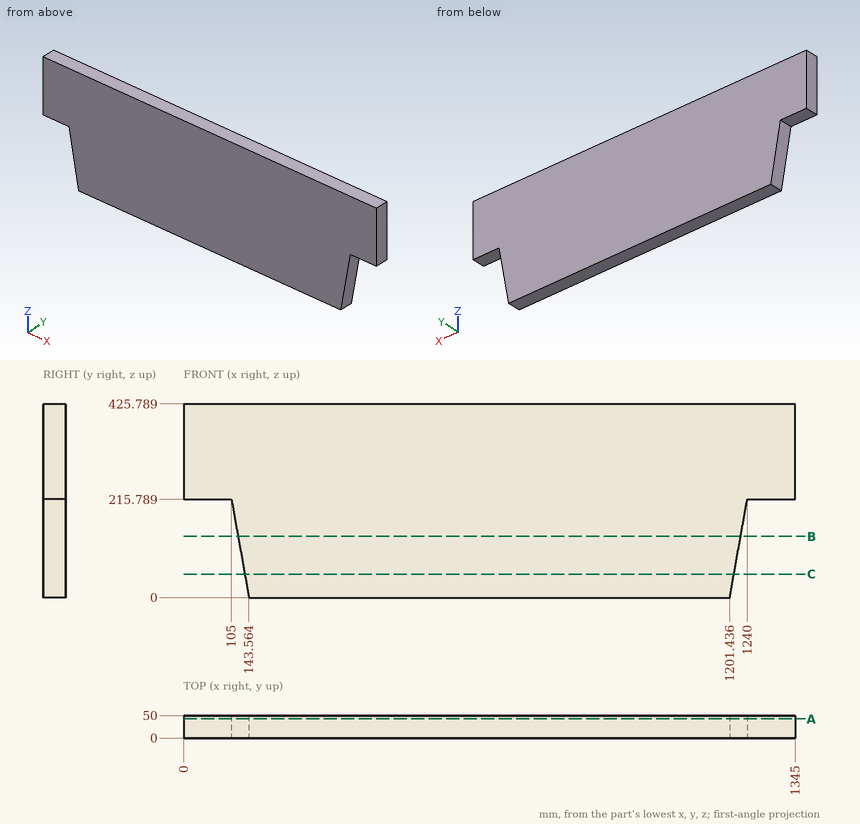
Geometry check sheet. Reference: drawing and pictorial views, mm from the part's lowest x, y, z. Give positions to 0.01 mm unless a question says otherwise; leave off trailing zeros. Loops run counter-clockwise (first coordinate to the right, second up) from the corner with the lowest first, then second, coordinate; pieces in that order, holes last. Notation, with made-up numbers: (-10.5, -19.5) -> (41.5, -19.5) arc R18 ccw to (41.5, -1.5) -> close; hole circle Ø4 at (-4, 49). An arc over 180 degrees is marked (long way). Answer in a Markdown table with one row per item. Add a question column.
1) Cross-section at C-C on z = 51.5. Record the boundary of the cut face in (x, y).
2) Cross-section at A-A on y = 42.5. Record the boundary of the cut face in (x, z) (1 decimal).
3) Cross-section at B-B on z = 134.5. Record the boundary of the cut face in (x, y), and give its area (3 significant figures).
4) Material ranges on probe 1 along Z at (x, y) = (87, 2); probe 2 along X at (y, z) = (34, 24) (1 decimal); probe 3 along X at (y, z) = (18.5, 93), recorded low to high. Write a range as from..to.
5) Gauge pin test, flat ends, axial feed: P1, Ø10, axis at y = 33, z = 86, coming from the +X side; P2, Ø15, axis at x = 1307.5, y = 16.5, coming from the -Z side. Record the tip position at first contact, or that the pin passes through.
Outcome:
| question | item | result |
|---|---|---|
| 1 | outline | (134.36, 0) -> (1210.64, 0) -> (1210.64, 50) -> (134.36, 50) -> close |
| 2 | outline | (0, 215.8) -> (105, 215.8) -> (143.6, 0) -> (1201.4, 0) -> (1240, 215.8) -> (1345, 215.8) -> (1345, 425.8) -> (0, 425.8) -> close |
| 3 | outline | (119.53, 0) -> (1225.47, 0) -> (1225.47, 50) -> (119.53, 50) -> close |
| 3 | area | 55,300 mm^2 |
| 4 | probe 1 | z = 215.79..425.79 |
| 4 | probe 2 | x = 139.3..1205.7 |
| 4 | probe 3 | x = 126.94..1218.06 |
| 5 | P1 | stops at x = 1217.7 |
| 5 | P2 | stops at z = 215.79 |
